```python
from build123d import *

# Parameters (mm, degrees)
SKETCH1_R           = 9.5
SKETCH1_R_2         = 3
BOSS_EXTRUDE1_DEPTH = 6
SKETCH2_R           = 5.2
SKETCH2_R_2         = 5
CUT_EXTRUDE1_DEPTH  = 0.2
SKETCH3_R           = 8.5
SKETCH3_R_2         = 7.85
CUT_EXTRUDE2_DEPTH  = 0.25
FILLET1_R           = 0.3
FILLET2_R           = 0.25


with BuildPart() as part:
    # Sketch1 → Boss-Extrude1 (new body)
    with BuildSketch(Plane.XY):
        Circle(SKETCH1_R)
        Circle(SKETCH1_R_2, mode=Mode.SUBTRACT)
    extrude(amount=BOSS_EXTRUDE1_DEPTH)

    # Sketch2 → Cut-Extrude1 (cut)
    with BuildSketch(Plane.XY.offset(6)):
        Circle(SKETCH2_R)
        Circle(SKETCH2_R_2, mode=Mode.SUBTRACT)
    cut_extrude1 = extrude(amount=-CUT_EXTRUDE1_DEPTH, mode=Mode.SUBTRACT)

    # Sketch3 → Cut-Extrude2 (cut)
    with BuildSketch(Plane.XY.offset(6)):
        Circle(SKETCH3_R)
        Circle(SKETCH3_R_2, mode=Mode.SUBTRACT)
    cut_extrude2 = extrude(amount=-CUT_EXTRUDE2_DEPTH, mode=Mode.SUBTRACT)

    # Mirror1: Cut-Extrude1, Cut-Extrude2 across plane
    add(cut_extrude1.mirror(Plane.XY.offset(3)), mode=Mode.SUBTRACT)
    add(cut_extrude2.mirror(Plane.XY.offset(3)), mode=Mode.SUBTRACT)

    # Fillet1
    fillet1_edges = [part.edges().sort_by_distance(p)[0] for p in [
        (-9.5, 0, 0),
        (-9.5, 0, 6),
    ]]
    fillet(fillet1_edges, radius=FILLET1_R)

    # Fillet2
    fillet2_edges = [part.edges().sort_by_distance(p)[0] for p in [
        (-3, 0, 0),
        (-3, 0, 6),
    ]]
    fillet(fillet2_edges, radius=FILLET2_R)


solid = part.part
```
Geometry check sheet. Reference: the model listing, model coordinates, mm. A direction names the side the tool comes from. Give positions to 0.01 mm unless a question says otherwise; leave off trailing zeros. Order: outer loops, then holes, each group sorted by start corner. A loop starts at its lowest first (then second) coordinate and runs counter-clockwise, first axis right, second up. Notation, with made-up numbers: (56, -21.75) - (115, -21.75) arc R20 cw to (115, 7.25) - close; hole circle Ø9 at (-19.5, -39). An arc over 180 degrees is marked (long way). Answer in a Markdown table with one row per item. Add a question column.
Q1. Gauge pin test, flat ends, axial feed: pin 1 (8 mm diameter, centred on x = 7, y = 4, fed in from +Z); pin 2 (1 mm diameter, centred on y = 3.5, z = 5.5, fed in from +X); pin 3 (3 mm diameter, centred on x = -5, z = 2, fed in from -Y); pin 4 (1 mm diameter, centred on y = 1.5, z = 2, fed in from +X). Record the tip position at first contact, or that the pin passes through.
Q2. Cross-section at A-A, the plane z = 4.55. Enter the section's corners in (x, y), then the cut area to 3 significant figures.
Q3. Mould release check, pull along Y, two halves, no side actions. Record for faces 1 (the flat face through (8, -2, 0.25)), 2 (the cylindrical face through (4.38, -8.43, 2.96)), 3 (the flat face through (5.4, -6.8, 0)): pulls with the +Y half, pulls with the -Y half, needs draft (parallel to the pull), parting line crosses it, or undercut.
Q4. Material ranges on probe 1 along Y at (x, z) = (0, 5.95); probe 2 along Y at (x, z) = (0, 0.15); probe 3 along Y at (x, z) = (0, 4.1), recorded low to high. Write a range as from..to.
Q5. Tool access check on faces 4 (the flat face through (3.3, -1, 0)), 5 (the flat face through (8, -2, 5.75)). Record the directions out of +Z, -Z, +X, -X, +Y, -Y that give a thin tool (end or side, any length) a straight path to the whole face; none if there is none.
Check values:
| question | item | result |
|---|---|---|
| 1 | pin 1 | stops at z = 6 |
| 1 | pin 2 | stops at x = 9.01 |
| 1 | pin 3 | stops at y = -8.83 |
| 1 | pin 4 | stops at x = 9.45 |
| 2 | outline | circle Ø19 at (0, 0); hole circle Ø6 at (0, 0) |
| 2 | area | 255 mm^2 |
| 3 | face 1 | undercut |
| 3 | face 2 | parting line crosses it |
| 3 | face 3 | needs draft |
| 4 | probe 1 | y = -9.37..-8.5, -7.85..-5.2, -5..-3.1, 3.1..5, 5.2..7.85, 8.5..9.37 |
| 4 | probe 2 | y = -9.46..-8.5, -7.85..-5.2, -5..-3.02, 3.02..5, 5.2..7.85, 8.5..9.46 |
| 4 | probe 3 | y = -9.5..-3, 3..9.5 |
| 5 | face 4 | -Z, +X, -X, +Y, -Y |
| 5 | face 5 | +Z |
